Input: part model. Units: mm. Frame: model coordinates. Coordinates: 2 decimals unless noted, no trailing zeros. Write each loop counter-clockwise with the first axis right and the second up, starting at its lowest first coordinate (ties: lowest second). Pieces come first, ordered by that corner, then holes. Notation, with made-up numbers: M -15,-7 L -11,-7 A18 ccw -11,7 Z; hole C 30.25,11.5 d1. An arc over 180 degrees is marked long. Write each question's results on one line, items separated by ' | '. Start each with the question number.
1. First-contact query: pin 1 (3 mm diameter, centred on x = 13, y = 17.5, fed in from -Z); pin 2 (2 mm diameter, centred on x = 39.5, z = 2, fed in from -Y); pin 3 (4 mm diameter, centred on y = 14, z = -6, fed in from -X). Flat tips, straight axial feed; report the tip coordinate or a pass-through.
2. Pull-direction query (Z, two-part tool) for faces 1 (the flat face through (35, 18.927, 12)), 2 (the cylindrical face through (39.853, 17.786, -0.66)), 3 (the cylindrical face through (5.79, 14.37, -6.01)); classes: +Z half, -Z half, draft (parallel to the pull), parting line (faces both ways), or undercut.
3. Ray query, probe 1 along X at (y, z) = (10.45, 0); probe 2 along X at (y, z) = (15.5, 5.5); probe 3 along Y at (x, z) = (21, 15.5). Return the intervals inside material, ascending.
4. Section query B-B, the plane y = 13.5. Output: boundary loops of the cut face in (x, z).
5. Section query A-A, the plane z = 0. Output: boundary loops of the cut face in (x, y).
```python
from build123d import *

# Parameters (mm, degrees)
F2_R = 0.4


with BuildPart() as f1:
    # F0 (on Top) → F1 (revolve)
    with BuildSketch(Plane.XY):
        with BuildLine():
            Line((4.8672996052, 18.9265990148), (4.8672996052, 9.9265990148))
            Line((4.8672996052, 9.9265990148), (9.3672996052, 9.9265990148))
            Line((9.3672996052, 9.9265990148), (9.8672996052, 9.9265990148))
            Line((9.8672996052, 9.9265990148), (9.8672996052, 12.2409004436))
            ThreePointArc((9.8672996052, 12.2409004436), (8.1513611708, 14.4265990148), (9.8672996052, 16.612297586))
            Line((9.8672996052, 16.612297586), (9.8672996052, 18.9265990148))
            Line((9.8672996052, 18.9265990148), (4.8672996052, 18.9265990148))
        make_face()
    revolve(axis=Axis((24.8672996052, 14.4265990148, 0), (0, -1, 0)))

    # F2
    f2_edges = [f1.edges().sort_by_distance(p)[0] for p in [
        (44.8673, 18.926599, 0),
        (44.8673, 9.926599, 0),
    ]]
    fillet(f2_edges, radius=F2_R)


solid = f1.part
```
Answer:
1) pin 1: z = -17.1 | pin 2: y = 9.93 | pin 3: x = 5.27
2) face 1: draft | face 2: undercut | face 3: parting line
3) probe 1: 4.87 to 9.87, 39.87 to 44.87 | probe 2: 5.64 to 9.37, 40.36 to 44.1 | probe 3: 9.93 to 12.76, 16.1 to 18.93
4) outline: C 24.87,0 d40; hole C 24.87,0 d33.03
5) outline: M 4.87,10.33 A0.4 ccw 5.27,9.93 L 9.87,9.93 L 9.87,12.24 A2.25 cw 9.87,16.61 L 9.87,18.93 L 5.27,18.93 A0.4 ccw 4.87,18.53 Z; M 39.87,9.93 L 44.47,9.93 A0.4 ccw 44.87,10.33 L 44.87,18.53 A0.4 ccw 44.47,18.93 L 39.87,18.93 L 39.87,16.61 A2.25 cw 39.87,12.24 Z
